Part print with two shaded views. Sizes in mm from the minimum x, y, z corner. A direction names the side the tool comes from. Round coordinates to 2 decimals unless told otherwise and drop trailing zeros. Write each loop counter-clockwise with the first axis right and the second up, starting at its lowest first coordinate (ties: lowest second). Pieces come first, ordered by that corner, then holes.
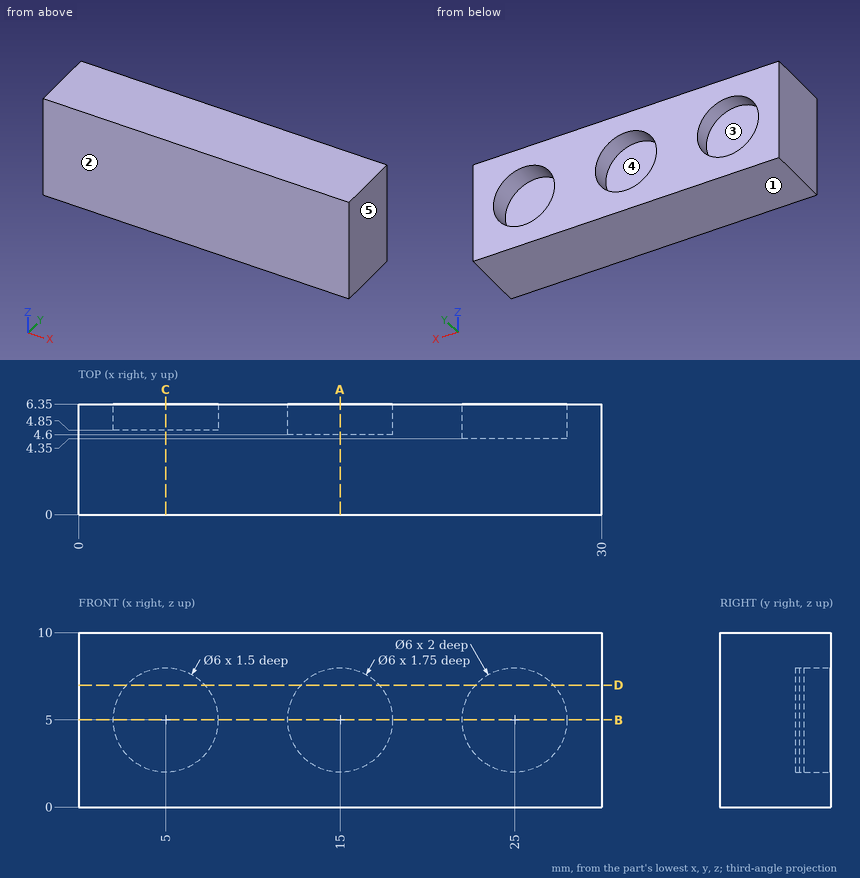
Q1. Wall check: L1, parallel to X at y = 4.8, z = 5; L2, parallel to X at y = 5.6, z = 5; L3, parallel to Z at x = 5, y = 6. Give the ranges that are in metal, low to high.
Values follow:
L1: x = 0 to 12, 18 to 22, 28 to 30
L2: x = 0 to 2, 8 to 12, 18 to 22, 28 to 30
L3: z = 0 to 2, 8 to 10
Q2. Which spindle directions (+Z, -Z, +X, -X, +Y, -Y) get a long thin tool onto all of the face, cutting with end or side? Do the marked faces 4 and 5. Say none if no direction does.
Values follow:
face 4: +Y
face 5: +Z, -Z, +X, +Y, -Y
Q3. Cut at D-D on z = 7. Write the cut outline in (x, y).
Values follow:
outline: (0, 0) - (30, 0) - (30, 6.35) - (27.24, 6.35) - (27.24, 4.35) - (22.76, 4.35) - (22.76, 6.35) - (17.24, 6.35) - (17.24, 4.6) - (12.76, 4.6) - (12.76, 6.35) - (7.24, 6.35) - (7.24, 4.85) - (2.76, 4.85) - (2.76, 6.35) - (0, 6.35) - close
Q4. Mould opens along Z. For the marked faces 1, 2 and 3 say: +Z half, -Z half, draft (parallel to the pull), parting line (faces both ways), or undercut.
Values follow:
face 1: -Z half
face 2: draft
face 3: undercut
Q5. Cut at A-A on x = 15. Write the cut outline in (y, z).
Values follow:
outline: (0, 0) - (6.35, 0) - (6.35, 2) - (4.6, 2) - (4.6, 8) - (6.35, 8) - (6.35, 10) - (0, 10) - close
Q6. Cut at B-B on z = 5. Write the cut outline in (x, y), plus the area to 3 significant figures.
Values follow:
outline: (0, 0) - (30, 0) - (30, 6.35) - (28, 6.35) - (28, 4.35) - (22, 4.35) - (22, 6.35) - (18, 6.35) - (18, 4.6) - (12, 4.6) - (12, 6.35) - (8, 6.35) - (8, 4.85) - (2, 4.85) - (2, 6.35) - (0, 6.35) - close
area: 159 mm2
Q7. Cut at C-C on x = 5. Write the cut outline in (y, z), plus the area to 3 significant figures.
Values follow:
outline: (0, 0) - (6.35, 0) - (6.35, 2) - (4.85, 2) - (4.85, 8) - (6.35, 8) - (6.35, 10) - (0, 10) - close
area: 54.5 mm2
Q8. Drop a flat-ended pin along its axis: pin 1 (5 mm diameter, centred on x = 25, z = 5, fed in from +Y). Give the stop position or say it passes through.
Values follow:
pin 1: stops at y = 4.35
